Drawing for the job (mm, zero at the part's lowest x, y, z). A direction names the side the tool comes from. Give positions to 0.01 mm unless a question says otherwise; leave off trailing zeros. Loops run counter-clockwise (first coordinate to the right, second up) from the corner with the lowest first, then second, coordinate; pieces in that order, holes last. Notation, with made-up numbers: (12, 4.25) - (27, 4.25) arc R37 cw to (27, 40.25) - close; hole circle Ø9 at (45, 86). An arc over 180 degrees is marked (long way). Return JSON: item names as keys, results as strings. Group by question number.
1) Mould opens along X. For the marked faces 5, 6, 7 and 8 say: released by +X, released by -X, zero draft, split by the parting line, or undercut.
2) Slice it at B-B (y = 40). List the corners of the cut face in (x, z).
3) Drill centre lines: probe 1 along X at (y, z) = (85, 40) (1 decimal); probe 2 along Z at (x, y) = (39, 94); probe 3 along X at (y, z) = (29, 58.5) (1 decimal). Where is each one in solid material? Low to high. Write a range as from..to.
4) 3-axis set-ups, long thin cutter, end or side, ignore diameter. For the marked faces 1, 2, 3 and 4: which of +Z, -Z, +X, -X, +Y, -Y reach the whole face in a straight line?
5) Slice it at A-A (z = 40). List the corners of the cut face in (x, y).
6) Slice it at C-C (x = 57.5). List the corners of the cut face in (y, z) (1 decimal), and give its area (3 significant figures).
7) Slice it at D-D (y = 153). Count the separate pieces of the cut face and the enclosed holes in it, and give its area (3 significant figures).
8) Drop flat-ended pins along their axis: pin 1 (12 mm diameter, centred on y = 155, z = 19, fed in from -X); pin 2 (10 mm diameter, centred on x = 88, z = 53, fed in from +Y); pin 3 (6 mm diameter, centred on y = 84, z = 56, fed in from -X). Give the stop position or say it passes through.
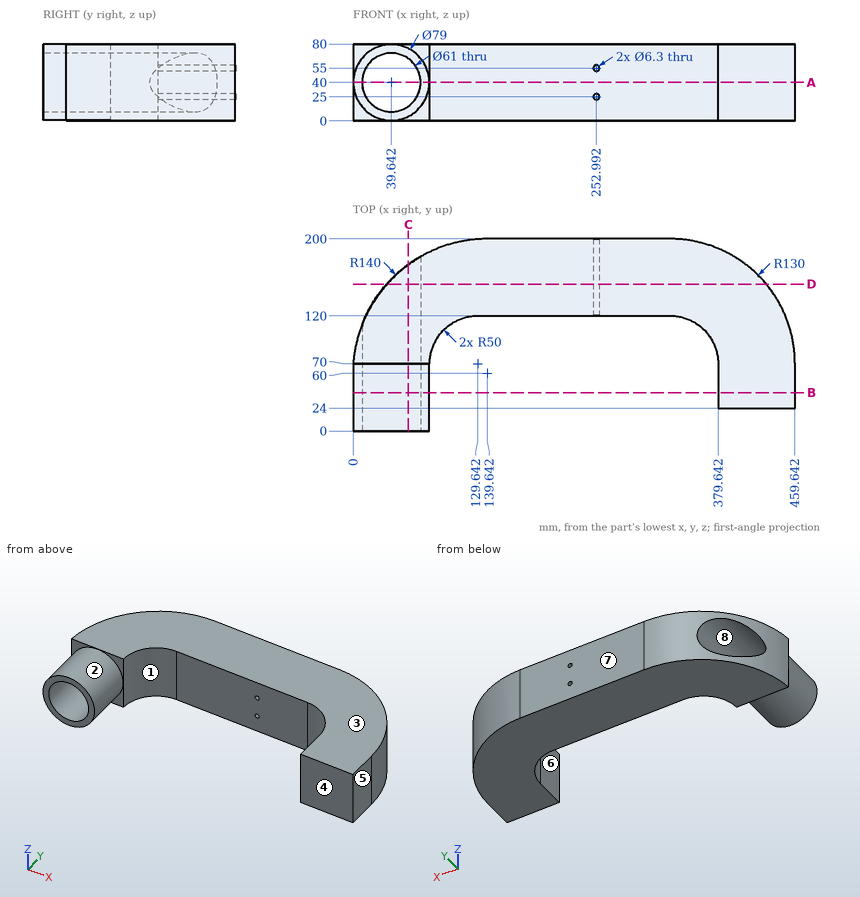
Results:
{
 "1": {"face 5": "released by +X", "face 6": "undercut", "face 7": "zero draft", "face 8": "undercut"},
 "2": {"outline": "circle Ø79 at (39.64, 40); (379.64, 0) - (459.64, 0) - (459.64, 80) - (379.64, 80) - close; hole circle Ø61 at (39.64, 40)"},
 "3": {"probe 1": "1.9..9.1, 70.1..81.9, 377.3..458.8", "probe 2": "0..9.51, 70.49..80", "probe 3": "4.7..15.4, 63.9..74.5, 379.6..459.6"},
 "4": {"face 1": "+Z, -Z, -Y", "face 2": "-Y", "face 3": "+Z, +X, -X, +Y, -Y", "face 4": "+Z, -Z, +X, -Y"},
 "5": {"outline": "(0, 70) - (0.14, 70) - (0.14, 0) - (9.14, 0) - (9.14, 110.69) arc R140 ccw to start; (70.14, 0) - (79.14, 0) - (79.14, 70) - (79.64, 70) arc R50 cw to (129.64, 120) - (329.64, 120) arc R50 cw to (379.64, 70) - (379.64, 24) - (459.64, 24) - (459.64, 70) arc R130 ccw to (329.64, 200) - (139.64, 200) arc R140 ccw to (70.14, 181.53) - close"},
 "6": {"outline": "(0, 4.8) - (70, 4.8) - (70, 0) - (173.4, 0) - (173.4, 15.3) - (0, 15.3) - close; (0, 64.7) - (173.4, 64.7) - (173.4, 80) - (70, 80) - (70, 75.2) - (0, 75.2) - close", "area": "4,630 mm2"},
 "7": {"separate pieces": "1", "enclosed holes": "2", "area": "29,800 mm2"},
 "8": {"pin 1": "x = 53.83", "pin 2": "y = 192", "pin 3": "x = 1.23"}
}
